CAD build for the part. Positions are in the model's coordinates, mm. Give positions to 0.01 mm unless a question says otherwise; leave off trailing zeros. Write each loop counter-clockwise with the first axis right and the second up, starting at its lowest first coordinate (ties: lowest second). Pieces come first, ordered by that corner, then holes. Notation, with made-up numbers: (80, 22.25) - (138, 22.25) arc R21 ccw to (138, 53.25) - close; hole circle Ø4 at (-21, 2.25). An arc over 180 degrees is marked (long way). Put each result on its own line as item: value. Start each with the question number.
1. Drop flat-ended pins along their axis: pin 1 (3 mm diameter, centred on x = -266, z = 3, fed in from -Y); pin 2 (2 mm diameter, centred on y = 55, z = 1, fed in from +X); pin 3 (1.5 mm diameter, centred on x = -267, z = 1, fed in from -Y). Give the stop position or say it passes through.
2. Cut at B-B on x = -269.5. List the corners of the cut face in (y, z) (3 decimals).
3. Mould opens along Y. For faces 1 (the flat face through (-254, 79, 3)), 2 (the flat face through (-253.02, 45.12, 3.13)), 3 (the flat face through (-247.456, 68.185, 3.131)), 4 (the flat face through (-260, 55, 0)) say: +Y half, -Y half, draft (parallel to the pull), parting line (faces both ways), or undercut.
4. Cut at C-C on y = 45.5. List the corners of the cut face in (x, z).
5. Cut at A-A on z = 1. Give the number of separate pieces and of enclosed holes in the cut face, and give its area (3 significant figures).
6. Wall check: line 1 (Y direction, x = -259, z = 0.5); line 2 (Y direction, x = -259.5, z = 6); line 3 (X direction, y = 63.5, z = 4.75). Give the ranges that are in metal, low to high.
from build123d import *

# Parameters (mm, degrees)
MODEL_R             = 1.925069784
BOSS_EXTRUDE1_DEPTH = 6.35


with BuildPart() as part:
    # Model → Boss-Extrude1 (new body)
    with BuildSketch(Plane.XY):
        with BuildLine():
            Line((-262.8855, 77.7663), (-272.8434, 36.5132))
            add(Edge.make_bspline(
                [(-272.8434, 36.5132), (-273.2663, 34.7494), (-272.1875, 32.9898), (-270.4236, 32.5666)],
                knots=[0.142857143, 0.142857143, 0.142857143, 0.142857143, 0.214285714, 0.214285714, 0.214285714, 0.214285714], degree=3))
            Line((-270.4236, 32.5666), (-260.0278, 30.0723))
            add(Edge.make_bspline(
                [(-260.0278, 30.0723), (-258.2636, 29.6496), (-256.5027, 30.7281), (-256.0795, 32.4923)],
                knots=[0.285714286, 0.285714286, 0.285714286, 0.285714286, 0.357142857, 0.357142857, 0.357142857, 0.357142857], degree=3))
            Line((-256.0795, 32.4923), (-249.8766, 58.0964))
            add(Edge.make_bspline(
                [(-249.8766, 58.0964), (-249.742, 58.0727), (-249.6054, 58.0619), (-249.4692, 58.0619)],
                knots=[0.428571429, 0.428571429, 0.428571429, 0.428571429, 0.5, 0.5, 0.5, 0.5], degree=3))
            add(Edge.make_bspline(
                [(-249.4692, 58.0619), (-248.1365, 58.0619), (-247.0559, 59.1417), (-247.0559, 60.4748)],
                knots=[0.5, 0.5, 0.5, 0.5, 0.571428571, 0.571428571, 0.571428571, 0.571428571], degree=3))
            add(Edge.make_bspline(
                [(-247.0559, 60.4748), (-247.0559, 61.5318), (-247.744, 62.4645), (-248.7524, 62.7785)],
                knots=[0.571428571, 0.571428571, 0.571428571, 0.571428571, 0.642857143, 0.642857143, 0.642857143, 0.642857143], degree=3))
            Line((-248.7524, 62.7785), (-246.1231, 73.7453))
            add(Edge.make_bspline(
                [(-246.1231, 73.7453), (-245.7003, 75.5091), (-246.7789, 77.27), (-248.5431, 77.6932)],
                knots=[0.714285714, 0.714285714, 0.714285714, 0.714285714, 0.785714286, 0.785714286, 0.785714286, 0.785714286], degree=3))
            Line((-248.5431, 77.6932), (-258.9389, 80.1862))
            add(Edge.make_bspline(
                [(-258.9389, 80.1862), (-259.1594, 80.2398), (-259.3787, 80.2689), (-259.5963, 80.2772)],
                knots=[0.857142857, 0.857142857, 0.857142857, 0.857142857, 1, 1, 1, 1], degree=3))
            add(Edge.make_bspline(
                [(-259.5963, 80.2772), (-261.1217, 80.3295), (-262.5167, 79.3095), (-262.8855, 77.7663)],
                knots=[0, 0, 0, 0, 0.071428571, 0.071428571, 0.071428571, 0.071428571], degree=3))
        make_face()
        with Locations((-254.25285, 72.3954)):
            Circle(MODEL_R, mode=Mode.SUBTRACT)
        with Locations((-259.47565, 52.9045)):
            Circle(MODEL_R, mode=Mode.SUBTRACT)
    extrude(amount=BOSS_EXTRUDE1_DEPTH)


solid = part.part
Report:
1. pin 1: stops at y = 31.15
1. pin 2: stops at x = -250.38
1. pin 3: stops at y = 31.57
2. outline: (32.345, 0) - (50.364, 0) - (50.364, 6.35) - (32.345, 6.35) - close
3. face 1: +Y half
3. face 2: -Y half
3. face 3: undercut
3. face 4: draft
4. outline: (-270.67, 0) - (-252.93, 0) - (-252.93, 6.35) - (-270.67, 6.35) - close
5. separate pieces: 1
5. enclosed holes: 2
5. area: 821 mm²
6. line 1: y = 29.99 to 51.04, 54.77 to 80.2
6. line 2: y = 29.99 to 50.98, 54.83 to 80.27
6. line 3: x = -266.33 to -248.58
